Work out the finished part from the listing and answer in its coordinate system (mm). Round coordinates to 2 decimals unless told otherwise and drop trailing zeros. Loops run counter-clockwise (first coordinate to the right, second up) from the corner with the lowest first, then second, coordinate; pieces in that order, holes last. Notation, with made-up numbers: (25, 81.25) -> (57, 81.25) arc R23 ccw to (57, 105.25) -> close; hole circle Ø7 at (84, 46.25). An arc over 180 degrees is marked (long way). Write item = value, one per line. Start each with the question number.
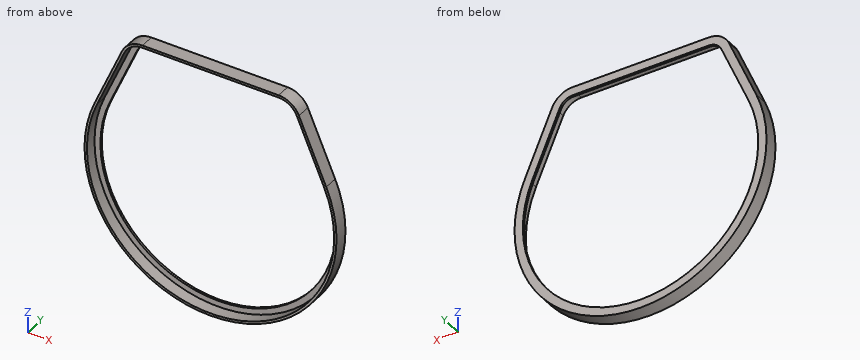
```python
from build123d import *

# Parameters (mm, degrees)
BOSS_EXTRUDE1_DEPTH = 6
BOSS_EXTRUDE2_DEPTH = 1.1


with BuildPart() as part:
    # Sketch1 → Boss-Extrude1 (new body)
    with BuildSketch(Plane(origin=(0, 0, 0), x_dir=(1, 0, 0), z_dir=(0, 1, 0))):
        with BuildLine():
            ThreePointArc((34.422746677, -63.95), (40.577345115, -62.107399108), (44.706859879, -57.185878226))
            Line((44.706859879, -57.185878226), (58.490893839, -25.229057412))
            ThreePointArc((58.490893839, -25.229057412), (0, 63.7), (-58.490893839, -25.229057412))
            Line((-58.490893839, -25.229057412), (-44.706859879, -57.185878226))
            ThreePointArc((-44.706859879, -57.185878226), (-40.577345115, -62.107399108), (-34.422746677, -63.95))
            Line((-34.422746677, -63.95), (34.422746677, -63.95))
        make_face()
        with BuildLine():
            Line((34.422746677, -62.75), (-34.422746677, -62.75))
            ThreePointArc((-34.422746677, -62.75), (-39.917923854, -61.104820632), (-43.604990608, -56.710605559))
            Line((-43.604990608, -56.710605559), (-57.389024568, -24.753784745))
            ThreePointArc((-57.389024568, -24.753784745), (-12.637957994, 61.208921063), (62.5, 0))
            ThreePointArc((62.5, 0), (61.208921063, -12.637957994), (57.389024568, -24.753784745))
            Line((57.389024568, -24.753784745), (43.604990608, -56.710605559))
            ThreePointArc((43.604990608, -56.710605559), (39.917923854, -61.104820632), (34.422746677, -62.75))
        make_face(mode=Mode.SUBTRACT)
    extrude(amount=BOSS_EXTRUDE1_DEPTH)

    # Sketch3 → Boss-Extrude2 (add)
    with BuildSketch(Plane(origin=(0, 6, 0), x_dir=(1, 0, 0), z_dir=(0, 1, 0))):
        with BuildLine():
            Line((-58.490893839, -25.229057412), (-44.706859879, -57.185878226))
            ThreePointArc((-44.706859879, -57.185878226), (-40.577345115, -62.107399108), (-34.422746677, -63.95))
            Line((-34.422746677, -63.95), (34.422746677, -63.95))
            ThreePointArc((34.422746677, -63.95), (40.577345115, -62.107399108), (44.706859879, -57.185878226))
            Line((44.706859879, -57.185878226), (58.490893839, -25.229057412))
            ThreePointArc((58.490893839, -25.229057412), (0, 63.7), (-58.490893839, -25.229057412))
        make_face()
        with BuildLine():
            Line((40.850317428, -55.522423891), (54.634351388, -23.565603077))
            ThreePointArc((54.634351388, -23.565603077), (0, 59.5), (-54.634351388, -23.565603077))
            Line((-54.634351388, -23.565603077), (-40.850317428, -55.522423891))
            ThreePointArc((-40.850317428, -55.522423891), (-38.269370701, -58.598374443), (-34.422746677, -59.75))
            Line((-34.422746677, -59.75), (34.422746677, -59.75))
            ThreePointArc((34.422746677, -59.75), (38.269370701, -58.598374443), (40.850317428, -55.522423891))
        make_face(mode=Mode.SUBTRACT)
    extrude(amount=BOSS_EXTRUDE2_DEPTH)


solid = part.part
```
Item 1: Flat-ended cylindrical pins translate along their axes: pin 1 (1.5 mm diameter, centred on x = -8, y = 6, fed in from -Z); pin 2 (1.5 mm diameter, centred on x = -48.5, z = 49, fed in from +Y); pin 3 (2 mm diameter, centred on y = 2.5, z = 38, fed in from +X). Find the tip coordinate at first contact, or state that the pin passes through.
Item 2: Section C-C (z = -16.5) is taken. Determine the outline of the cut face in (x, y).
Item 3: Section A-A (x = 0) is taken. Determine the outline of the cut face in (y, z), then the cut area to 3 significant figures.
Item 4: Section B-B (y = 3.25) is taken. Determine the outline of the cut face in (x, z) (3 decimals), then the cut area to 3 significant figures.
Item 5: Find the intervals of material crossed by line 1 along X through (y, z) = (2.85, 0); line 2 along Z through (x, y) = (-2, 6.75); line 3 along Z through (x, y) = (-0.5, 2), in increasing order. Write a range as [from, to].
Worked answers:
q1.pin_1 = -63.29
q1.pin_2 = 7.1
q1.pin_3 = 53.41
q2.outline = (-61.53, 0) -> (-60.28, 0) -> (-60.28, 6) -> (-57.17, 6) -> (-57.17, 7.1) -> (-61.53, 7.1) -> close; (57.17, 6) -> (60.28, 6) -> (60.28, 0) -> (61.53, 0) -> (61.53, 7.1) -> (57.17, 7.1) -> close
q3.outline = (0, -63.7) -> (7.1, -63.7) -> (7.1, -59.5) -> (6, -59.5) -> (6, -62.5) -> (0, -62.5) -> close; (0, 62.75) -> (6, 62.75) -> (6, 59.75) -> (7.1, 59.75) -> (7.1, 63.95) -> (0, 63.95) -> close
q3.area = 23.6 mm2
q4.outline = (-58.491, 25.229) arc R63.7 ccw (long way) to (58.491, 25.229) -> (44.707, 57.186) arc R11.2 ccw to (34.423, 63.95) -> (-34.423, 63.95) arc R11.2 ccw to (-44.707, 57.186) -> close; hole (-57.389, 24.754) arc R62.5 ccw (long way) to (57.389, 24.754) -> (43.605, 56.711) arc R10 ccw to (34.423, 62.75) -> (-34.423, 62.75) arc R10 ccw to (-43.605, 56.711) -> close
q4.area = 495 mm2
q5.line_1 = [-63.7, -62.5], [62.5, 63.7]
q5.line_2 = [-63.67, -59.47], [59.75, 63.95]
q5.line_3 = [-63.7, -62.5], [62.75, 63.95]
